Geometry: final body of the model. Coordinates: model frame, mm. Face numbers are marked on the shaded views. A direction names the side the tool comes from. Give positions to 0.01 mm unless a question says otherwise; leave off trailing zeros. Write each loop counter-clockwise with the first axis right and the second up, starting at its lowest first coordinate (ties: lowest second). Pieces come first, ordered by that corner, then holes. Notation, with made-up numbers: (-10, 18) -> (1, 18) arc R25 cw to (1, 53) -> close; hole circle Ø4 at (53.25, 80). An arc over 180 degrees is marked (long way). Answer as a JSON object with one key per item and string values.
from build123d import *

# Parameters (mm, degrees)
IZIM3_W                                          = 3.5
IZIM3_H                                          = 23
IZIM3_H_2                                        = 5
IZIM3_W_2                                        = 2.5
Y_KSEKLIK_EKSTR_ZYON3_DEPTH                      = 8.28
IZIM4_W                                          = 7
IZIM4_H                                          = 5.16
KES_EKSTR_ZYON1_DEPTH                            = 34
IZIM11_W                                         = 12
IZIM11_H                                         = 33
KES_EKSTR_ZYON2_DEPTH                            = 1
M2_D_Z_BA_L_MAKINE_VIDAS_IN_HAV_A_DE_D           = 2.2
M2_D_Z_BA_L_MAKINE_VIDAS_IN_HAV_A_DE_CSINK_D     = 2.6
M2_D_Z_BA_L_MAKINE_VIDAS_IN_HAV_A_DE_CSINK_ANGLE = 90
IZIM16_W                                         = 12
IZIM16_H                                         = 33
KES_EKSTR_ZYON3_DEPTH                            = 10


with BuildPart() as part:
    # Çizim3 → Yükseklik-Ekstrüzyon3 (new body)
    with BuildSketch(Plane(origin=(0, 0, 0), x_dir=(1, 0, 0), z_dir=(0, 1, 0))):
        with BuildLine():
            Line((16, 6.5), (16, 11.5))
            Line((16, 11.5), (11.324751653, 11.5))
            ThreePointArc((11.324751653, 11.5), (10.819882158, 9.603828792), (10, 7.821091654))
            Line((10, 7.821091654), (10, -21.5))
            Line((10, -21.5), (16, -21.5))
            Line((16, -21.5), (16, -16.5))
            Line((16, -16.5), (16, 6.5))
        make_face()
        with Locations((17.75, -5)):
            Rectangle(IZIM3_W, IZIM3_H)
        with Locations((17.75, 9)):
            Rectangle(IZIM3_W, IZIM3_H_2)
        with Locations((20.75, 9)):
            Rectangle(IZIM3_W_2, IZIM3_H_2)
        with Locations((17.75, -19)):
            Rectangle(IZIM3_W, IZIM3_H_2)
        with Locations((20.75, -19)):
            Rectangle(IZIM3_W_2, IZIM3_H_2)
    y_kseklik_ekstr_zyon3 = extrude(amount=Y_KSEKLIK_EKSTR_ZYON3_DEPTH)

    # Çizim4 → Kes-Ekstrüzyon1 (cut, through all)
    with BuildSketch(Plane.XY.offset(21.5)):
        with Locations((13.5, 2.58)):
            Rectangle(IZIM4_W, IZIM4_H)
    kes_ekstr_zyon1 = extrude(amount=-KES_EKSTR_ZYON1_DEPTH, mode=Mode.SUBTRACT)

    # Çizim11 → Kes-Ekstrüzyon2 (cut)
    with BuildSketch(Plane(origin=(0, 8.28, 0), x_dir=(1, 0, 0), z_dir=(0, 1, 0))):
        with Locations((16, -5)):
            Rectangle(IZIM11_W, IZIM11_H)
    kes_ekstr_zyon2 = extrude(amount=-KES_EKSTR_ZYON2_DEPTH, mode=Mode.SUBTRACT)

    # M2 Düz Başlı Makine Vidası İçin Havşa_ DEĞİŞTİREBİLİRİZ (through all)
    with Locations(Plane(origin=(19.5, 7.28, 19), x_dir=(0, 0, 1), z_dir=(0, 1, 0))):
        with Locations((0, 0), (-28, 0), (-2, -6), (-10, -6), (-18, -6), (-26, -6)):
            m2_d_z_ba_l_makine_vidas_in_hav_a_de = CounterSinkHole(M2_D_Z_BA_L_MAKINE_VIDAS_IN_HAV_A_DE_D / 2, M2_D_Z_BA_L_MAKINE_VIDAS_IN_HAV_A_DE_CSINK_D / 2, counter_sink_angle=M2_D_Z_BA_L_MAKINE_VIDAS_IN_HAV_A_DE_CSINK_ANGLE)

    # Aynalama2: Yükseklik-Ekstrüzyon3, Kes-Ekstrüzyon1, Kes-Ekstrüzyon2, M2 Düz Başlı Makine Vidası İçin Havşa_ DEĞİŞTİREBİLİRİZ across plane
    add(y_kseklik_ekstr_zyon3.mirror(Plane(origin=(10, 8.28, 0), x_dir=(0, 0, 1), z_dir=(-1, 0, 0))))
    add(kes_ekstr_zyon1.mirror(Plane(origin=(10, 8.28, 0), x_dir=(0, 0, 1), z_dir=(-1, 0, 0))), mode=Mode.SUBTRACT)
    add(kes_ekstr_zyon2.mirror(Plane(origin=(10, 8.28, 0), x_dir=(0, 0, 1), z_dir=(-1, 0, 0))), mode=Mode.SUBTRACT)
    add(m2_d_z_ba_l_makine_vidas_in_hav_a_de.mirror(Plane(origin=(10, 8.28, 0), x_dir=(0, 0, 1), z_dir=(-1, 0, 0))), mode=Mode.SUBTRACT)

    # Çizim16 → Kes-Ekstrüzyon3 (cut)
    with BuildSketch(Plane(origin=(0, 7.28, 0), x_dir=(1, 0, 0), z_dir=(0, 1, 0))):
        with Locations((16, -5)):
            Rectangle(IZIM16_W, IZIM16_H)
    extrude(amount=-KES_EKSTR_ZYON3_DEPTH, mode=Mode.SUBTRACT)


solid = part.part
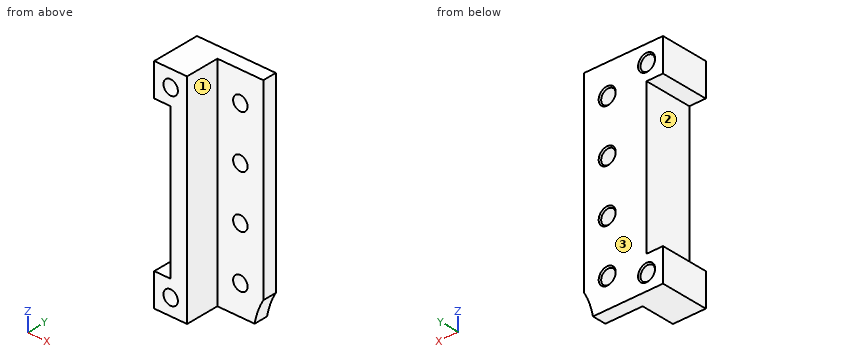
Q1. Cut plane B-B (z = 1). Return the cut outline in (x, y).
Values:
{"outline": "(0.5, 0) -> (3, 0) -> (3, 5.16) -> (5.4, 5.16) -> (5.4, 7.08) -> (5.2, 7.28) -> (0.5, 7.28) -> close; (7.6, 5.16) -> (10, 5.16) -> (10, 7.28) -> (7.8, 7.28) -> (7.6, 7.08) -> close"}
Q2. Cut plane D-D (z = -7). Return the cut outline in (x, y), and give its area (3 significant figures).
Values:
{"outline": "(-2, 0) -> (3, 0) -> (3, 5.16) -> (5.4, 5.16) -> (5.4, 7.08) -> (5.2, 7.28) -> (-2, 7.28) -> close; (7.6, 5.16) -> (10, 5.16) -> (10, 7.28) -> (7.8, 7.28) -> (7.6, 7.08) -> close", "area": "46.5 mm²"}
Q3. Cut plane A-A (x = 6.5). Return the cut outline in (y, z).
Values:
{"outline": "(5.16, -11.5) -> (7.28, -11.5) -> (7.28, -8.3) -> (7.08, -8.1) -> (5.16, -8.1) -> close; (5.16, -5.9) -> (7.08, -5.9) -> (7.28, -5.7) -> (7.28, -0.3) -> (7.08, -0.1) -> (5.16, -0.1) -> close; (5.16, 2.1) -> (7.08, 2.1) -> (7.28, 2.3) -> (7.28, 7.7) -> (7.08, 7.9) -> (5.16, 7.9) -> close; (5.16, 10.1) -> (7.08, 10.1) -> (7.28, 10.3) -> (7.28, 15.7) -> (7.08, 15.9) -> (5.16, 15.9) -> close; (5.16, 18.1) -> (7.08, 18.1) -> (7.28, 18.3) -> (7.28, 21.5) -> (5.16, 21.5) -> close"}
Q4. First-contact query: P1, Ø2, axis at x = 7.5, z = 7.5, coming from the -Y side; P2, Ø3.5, axis at y = 2, z = 8.5, coming from the -X side. Flat tips, straight axial feed; report the tip coordinate or a pass-through.
Values:
{"P1": "y = 5.16", "P2": "x = 0.5"}
Q5. Set-up query: the marked faces 1, 2 and 3. Return all of +Z, -Z, +X, -X, +Y, -Y with unobstructed straight access to the full face (end or side cutting, diameter ignored); none if empty.
Values:
{"face 1": "+Z, -Z, +X, -Y", "face 2": "-X, +Y, -Y", "face 3": "+Z, -Z, +X, -X, +Y"}
Q6. Cut plane C-C (y = 3). Return the cut outline in (x, z), and give its area (3 significant figures).
Values:
{"outline": "(-2, -11.5) -> (3, -11.5) -> (3, 21.5) -> (-2, 21.5) -> (-2, 16.5) -> (0.5, 16.5) -> (0.5, -6.5) -> (-2, -6.5) -> close; hole circle Ø2.2 at (0.5, -9); hole circle Ø2.2 at (0.5, 19)", "area": "99.9 mm²"}
Q7. Material intervals for L1, parallel to Z at x = 0.25, y = 5.75; L2, parallel to X at y = 4, z = 19; L3, parallel to X at y = 6.75, z = -7, sorted ascending. Write a range as from..to.
Values:
{"L1": "-11.5..-10.07, -7.93..-6.5, 16.5..17.93, 20.07..21.5", "L2": "-2..-0.6, 1.6..3", "L3": "-2..5.4, 7.6..10"}
